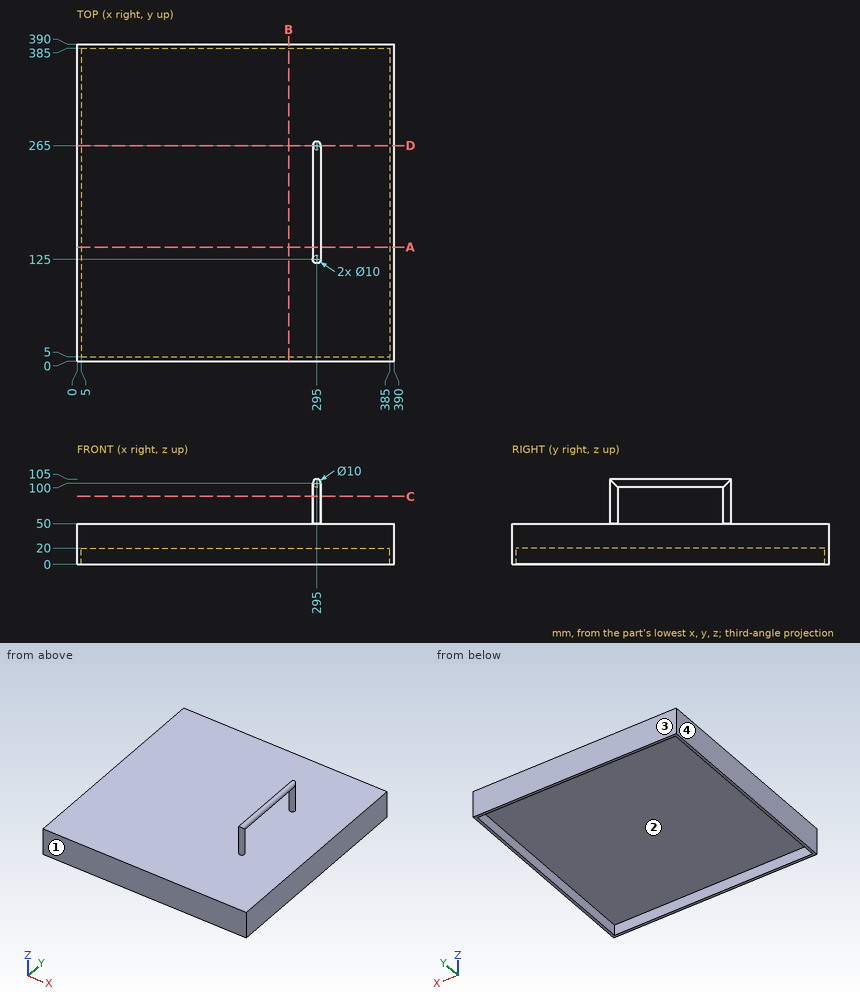
Answer from the drawing. Dimensions are ordinates in mm from the lowest x, y and z of the part. Round coordinates to 2 decimals unless told otherwise and drop trailing zeros. Loops run counter-clockwise (first coordinate to the right, second up) from the corner with the lowest first, then second, coordinate; pieces in that order, holes last. Notation, with made-up numbers: (53.25, 9.25) - (106.25, 9.25) arc R15 cw to (106.25, 22.25) - close; hole circle Ø10 at (60.25, -1). An arc over 180 degrees is marked (long way). Return JSON: item names as keys, results as strings. Group by question number.
1. The part is cut by section A-A on y = 140. Determine the outline of the cut face in (x, z), then the cut area to 3 significant figures.
2. Consider probe 1 along Y at (x, z) = (356, 15); probe 2 along Z at (x, y) = (183.5, 139.5). Determine where each line is inside the solid, lowest interval first.
3. The part is cut by section D-D on y = 265. Determine the outline of the cut face in (x, z), then the cut area to 3 significant figures.
4. The part is cut by section B-B on x = 260.5. Determine the outline of the cut face in (y, z), then the cut area to 3 significant figures.
5. The part is cut by section C-C on z = 83.5. Determine the outline of the cut face in (x, y), then the cut area to 3 significant figures.
6. The mould has two halves that part along Y. Classify the marked faces 1, 2, 3 and 4: pulls with the +Y half, pulls with the -Y half, needs draft (parallel to the pull), parting line crosses it, or undercut.
7. Each of these flat-tipped pins is pushed along its axis until it touches: P1, Ø12, axis at x = 116.5, y = 272, coming from the -Z side; P2, Ø5, axis at x = 89.5, y = 295.5, coming from the +Z side. Where does it stop, or does it pass through?
Resolved:
{
 "1": {"outline": "(0, 0) - (5, 0) - (5, 20) - (385, 20) - (385, 0) - (390, 0) - (390, 50) - (0, 50) - close; circle Ø10 at (295, 100)", "area": "12,000 mm²"},
 "2": {"probe 1": "y = 0 to 5, 385 to 390", "probe 2": "z = 20 to 50"},
 "3": {"outline": "(0, 0) - (5, 0) - (5, 20) - (385, 20) - (385, 0) - (390, 0) - (390, 50) - (300, 50) - (300, 100) arc R5 ccw to (290, 100) - (290, 50) - (0, 50) - close", "area": "12,400 mm²"},
 "4": {"outline": "(0, 0) - (5, 0) - (5, 20) - (385, 20) - (385, 0) - (390, 0) - (390, 50) - (0, 50) - close", "area": "11,900 mm²"},
 "5": {"outline": "circle Ø10 at (295, 125); circle Ø10 at (295, 265)", "area": "157 mm²"},
 "6": {"face 1": "pulls with the -Y half", "face 2": "undercut", "face 3": "pulls with the +Y half", "face 4": "needs draft"},
 "7": {"P1": "stops at z = 20", "P2": "stops at z = 50"}
}
